Check sheet for the modelled part. Datum: model origin and axes. Units: mm. Give positions to 0.01 mm unless a question says otherwise; leave off trailing zeros. Answer as CSV lines item,"result". Start each with the question number.
(1) Gauge pin test, flat ends, axial feed: pin 1 Ø6 at (x, z) = (6.5, 2.5) entering from +Y; pin 2 Ø3 at (y, z) = (-226.5, -2) entering from -X; pin 3 Ø1.5 at (x, z) = (-5.5, -9.5) entering from -Y; pin 4 Ø1.1 at (x, y) = (2, -281.5) entering from +Z. Record the tip position at first contact, or that the pin passes through.
(2) Section check A-A on y = -327.5. State how many separate pieces and enclosed holes the cut face has, plus the area to 3 significant figures.
(3) Material ranges on line 1 (X direction, y = -354.5, z = -12.5); line 2 (X direction, y = -74, z = 13.25), recorded low to high. Write a range as from..to.
from build123d import *

# Parameters (mm, degrees)
F0_W     = 4
F0_H     = 4
F1_DEPTH = 400
F2_R     = 0.2


# Not quite as in the source:
# - ends of sketch curves that miss each other by under 0.0002 mm in the source are joined


with BuildPart() as f1:
    # F0 (on Front) → F1 (new body)
    with BuildSketch(Plane.XZ):
        Polygon((-4, 12.7), (-4, 15), (-15, 15), (-15, 4), (-12.7, 4), (-12.7, 8.4000005318), (-10.2000002146, 8.4000002226), (-5.9999986286, 4.1999975978), (-5.9999986286, 0.5), (-5.4999986286, 0), (-5.9999986286, -0.5), (-5.9999986286, -4.1999975978), (-10.2000002146, -8.4000002226), (-12.7, -8.4000005401), (-12.7, -4), (-15, -4), (-15, -15), (-4, -15), (-4, -12.7), (-8.4, -12.7), (-8.4, -10.1349351573), (-4.265066287, -6.0000004215), (-0.5, -6.0000004215), (0, -5.5000004215), (0.5, -6.0000004215), (4.265066287, -6.0000004215), (8.4, -10.1349351573), (8.4, -12.7), (4, -12.7), (4, -15), (15, -15), (15, -4), (12.7, -4), (12.7, -8.4000005318), (10.2000002146, -8.4000002143), (5.9999986286, -4.1999975978), (5.9999986286, -0.5), (5.4999986286, 0), (5.9999986286, 0.5), (5.9999986286, 4.1999975978), (10.2000002146, 8.4000002226), (12.7, 8.4000005318), (12.7, 4), (15, 4), (15, 15), (4, 15), (4, 12.7), (8.4, 12.7), (8.4, 10.1349351573), (4.265066287, 6.0000004215), (0.5, 6.0000004215), (0, 5.5000004215), (-0.5, 6.0000004215), (-4.265066287, 6.0000004215), (-8.4, 10.1349351573), (-8.4, 12.7), align=None)
        with Locations((-11.7, -11.7000005318)):
            Rectangle(F0_W, F0_H, mode=Mode.SUBTRACT)
        with Locations((11.7, -11.7000005318)):
            Rectangle(F0_W, F0_H, mode=Mode.SUBTRACT)
        with BuildLine():
            Line((-3.1892931549, 1.7750800467), (-4.6035065879, 3.1892937385))
            Line((-4.6035065879, 3.1892937385), (-3.896399742, 3.896400455))
            Line((-3.896399742, 3.896400455), (-3.1892928961, 4.6035071715))
            Line((-3.1892928961, 4.6035071715), (-1.7750794631, 3.1892934797))
            ThreePointArc((-1.7750794631, 3.1892934797), (-5.13e-08, 3.6466421089), (1.7750793605, 3.1892934797))
            Line((1.7750793605, 3.1892934797), (3.1892927707, 4.6035071942))
            Line((3.1892927707, 4.6035071942), (3.896399628, 3.8964004891))
            Line((3.896399628, 3.8964004891), (4.6035064852, 3.189293784))
            Line((4.6035064852, 3.189293784), (3.189293075, 1.7750800695))
            ThreePointArc((3.189293075, 1.7750800695), (3.6502008105, 3.145e-07), (3.189293075, -1.7750794404))
            Line((3.189293075, -1.7750794404), (4.6035060628, -3.1892944964))
            Line((4.6035060628, -3.1892944964), (3.8964005729, -3.8963996238))
            Line((3.8964005729, -3.8963996238), (3.1892938779, -4.6035064911))
            Line((3.1892938779, -4.6035064911), (1.775078938, -3.189293772))
            ThreePointArc((1.775078938, -3.189293772), (8.169e-07, -3.6522284465), (-1.775078938, -3.189293772))
            Line((-1.775078938, -3.189293772), (-3.1892921382, -4.6035076966))
            Line((-3.1892921382, -4.6035076966), (-3.8964003567, -3.8964000069))
            Line((-3.8964003567, -3.8964000069), (-4.6035070554, -3.1892931432))
            Line((-4.6035070554, -3.1892931432), (-3.1892931549, -1.7750794631))
            ThreePointArc((-3.1892931549, -1.7750794631), (-3.6388745209, 2.918e-07), (-3.1892931549, 1.7750800467))
        make_face(mode=Mode.SUBTRACT)
        with Locations((-11.7, 11.7000005318)):
            Rectangle(F0_W, F0_H, mode=Mode.SUBTRACT)
        with Locations((11.7, 11.7000005318)):
            Rectangle(F0_W, F0_H, mode=Mode.SUBTRACT)
    extrude(amount=F1_DEPTH)

    # F2
    f2_edges = [f1.edges().sort_by_distance(p)[0] for p in [
        (-4, -200, 15),
        (4, -200, 15),
        (-15, -200, 15),
        (15, -200, 15),
        (-12.7, -200, 4),
        (-15, -200, 4),
        (-15, -200, -4),
        (-15, -200, -15),
        (-4, -200, -15),
        (-4, -200, -12.7),
        (-12.7, -200, -4),
        (4, -200, -15),
        (15, -200, -15),
        (12.7, -200, -4),
        (12.7, -200, 4),
        (15, -200, -4),
        (15, -200, 4),
        (-4, -200, 12.7),
        (4, -200, -12.7),
        (4, -200, 12.7),
        (9.7, -200, 13.700001),
        (-13.7, -200, 13.700001),
        (-13.7, -200, -9.700001),
        (9.7, -200, -9.700001),
        (-9.7, -200, 9.700001),
        (-9.7, -200, -13.700001),
        (13.7, -200, -13.700001),
        (13.7, -200, 9.700001),
        (13.7, -200, 13.700001),
        (-9.7, -200, 13.700001),
        (-9.7, -200, -9.700001),
        (13.7, -200, -9.700001),
        (9.7, -200, 9.700001),
        (-13.7, -200, 9.700001),
        (9.7, -200, -13.700001),
        (-13.7, -200, -13.700001),
    ]]
    fillet(f2_edges, radius=F2_R)


solid = f1.part
Working result:
1,pin 1,"stops at y = 0"
1,pin 2,"stops at x = -6"
1,pin 3,"passes through"
1,pin 4,"stops at z = 6"
2,separate pieces,"1"
2,enclosed holes,"5"
2,area,"324 mm^2"
3,line 1,"x = -15..-13.7, -9.7..-8.4, 8.4..9.7, 13.7..15"
3,line 2,"x = -15..-13.7, -9.7..-4, 4..9.7, 13.7..15"
